```python
from build123d import *

# Parameters (mm, degrees)
SKETCH2_R           = 7.5
BOSS_EXTRUDE1_DEPTH = 15
SKETCH3_R           = 6.5
BOSS_EXTRUDE2_DEPTH = 7.5
SKETCH4_R           = 11
BOSS_EXTRUDE3_DEPTH = 15
SKETCH5_R           = 20
CUT_EXTRUDE1_DEPTH  = 235


with BuildPart() as part:
    # Sketch1 → Revolve1 (revolve)
    with BuildSketch(Plane.XY, mode=Mode.PRIVATE) as revolve1_sk:
        Polygon((0, 0), (35, 0), (35, 50), (30, 50), (30, 130), (35, 130), (35, 180), (22.65711135, 250), (30, 250), (30, 260), (0, 260), align=None)
    revolve(revolve1_sk.sketch.rotate(Axis((0, 0, 0), (0, 1, 0)), 90), axis=Axis((0, 0, 0), (0, 1, 0)))

    # Sketch2 → Boss-Extrude1 (add)
    with BuildSketch(Plane.XY.offset(35)):
        with BuildLine():
            Line((0, 0), (48, 0))
            Line((48, 0), (65, 0))
            ThreePointArc((65, 0), (79.305754261, 10.489413007), (73.603646545, 27.287280664))
            Line((73.603646545, 27.287280664), (41.166521698, 50))
            Line((41.166521698, 50), (0, 50))
            Line((0, 50), (0, 0))
        make_face()
        with Locations((48, 19)):
            Circle(SKETCH2_R, mode=Mode.SUBTRACT)
    boss_extrude1 = extrude(amount=-BOSS_EXTRUDE1_DEPTH)

    # Mirror1: Boss-Extrude1 across plane
    add(boss_extrude1.mirror(Plane.XY))

    # Sketch3 → Boss-Extrude2 (add, symmetric)
    with BuildSketch(Plane.XY):
        with BuildLine():
            Line((0, 180), (0, 140.71))
            Line((0, 140.71), (55, 140.71))
            Line((55, 140.71), (60, 140.71))
            ThreePointArc((60, 140.71), (71.563565439, 149.503139487), (66.180456899, 162.996007608))
            Line((66.180456899, 162.996007608), (37.881061244, 180))
            Line((37.881061244, 180), (0, 180))
        make_face()
        with Locations((55, 155)):
            Circle(SKETCH3_R, mode=Mode.SUBTRACT)
    boss_extrude2 = extrude(amount=BOSS_EXTRUDE2_DEPTH, both=True)

    # Mirror2: Boss-Extrude2 across plane
    add(boss_extrude2.mirror(Plane(origin=(0, 0, 0), x_dir=(0, 0, 1), z_dir=(1, 0, 0))))

    # Sketch4 → Boss-Extrude3 (add)
    with BuildSketch(Plane.XY.offset(5)):
        with BuildLine():
            Line((-20, 290), (-20, 258.467022151))
            Line((-20, 258.467022151), (20, 258.467022151))
            Line((20, 258.467022151), (20, 290))
            ThreePointArc((20, 290), (0, 310), (-20, 290))
        make_face()
        with Locations((0, 290)):
            Circle(SKETCH4_R, mode=Mode.SUBTRACT)
    extrude(amount=BOSS_EXTRUDE3_DEPTH)

    # Sketch5 → Cut-Extrude1 (cut)
    with BuildSketch(Plane.XZ):
        with Locations(Location((0, 0, 0), (0, 0, 270))):
            Circle(SKETCH5_R)
    extrude(amount=-CUT_EXTRUDE1_DEPTH, mode=Mode.SUBTRACT)


solid = part.part
```
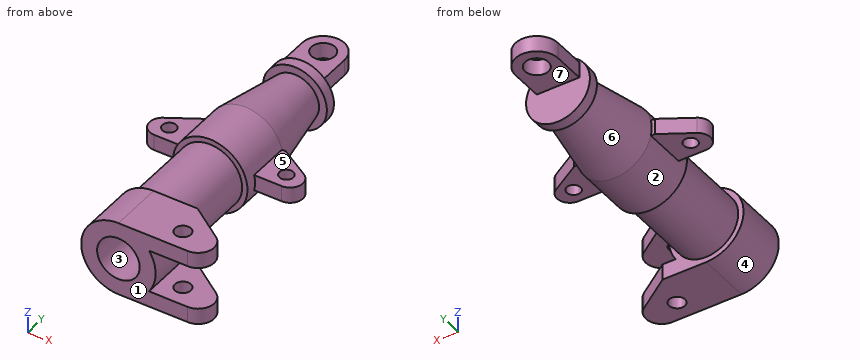
The listing builds one solid part. Answer for the finished solid, in the listing's coordinates (mm). Face numbers are marked on the shaded views. A direction names the side the tool comes from. Coordinates: 2 decimals unless noted, no trailing zeros. Loops run counter-clockwise (first coordinate to the right, second up) from the corner with the lowest first, then second, coordinate; pieces in that order, holes last. Notation, with made-up numbers: M -15,14 L 44,14 A28 cw 44,33 Z; hole C -25.75,71.5 d11. An arc over 180 degrees is marked long. Answer as a JSON object with one key per item and string values. Group by question number.
Item 1: Section C-C (y = 43) is taken. Write down the section's boundary in (x, z).
Item 2: Determine the mould class of the marked faces 1, 2, 3 and 4 for opening direction X: +X half, -X half, draft (parallel to the pull), parting line (faces both ways), or undercut.
Item 3: Which of the six approach directions +Z, -Z, +X, -X, +Y, -Y give full straight-line access (tool end or side, diameter ignored) to the marked faces 5, 6 and 7?
Item 4: Section D-D (z = -26.5) is taken. Give the number of separate pieces and of enclosed holes in the cut face, and give its area (3 significant figures).
Item 5: Each of these flat-tipped pins is pushed along its axis until it touches: P1, Ø1.1, axis at x = -35.5, z = 3.5, coming from the +Y side; P2, Ø5, axis at x = 38.5, y = 159.5, coming from the -Z side; P3, Ø10, axis at y = 209, z = 16, coming from the +X side. Where does it stop, or does it pass through?
Item 6: Section A-A (y = 155) is taken. Write down the section's boundary in (x, z).
Item 7: Section B-B (x = -55) is taken. Write down the section's boundary in (y, z).
Item 8: Consider L1, parallel to X at y = 93, z = 0; L2, parallel to Z at x = 11, y = 294.5; L3, parallel to X at y = 15, z = -23.5. Determine where each line is inside the solid, lowest interval first.
Solved:
{
 "1": {"outline": "M 0,-35 L 51.16,-35 L 51.16,-20 L 28.72,-20 A35 ccw 28.72,20 L 51.16,20 L 51.16,35 L 0,35 A35 ccw Z; hole C 0,0 d40"},
 "2": {"face 1": "draft", "face 2": "parting line", "face 3": "undercut", "face 4": "-X half"},
 "3": {"face 5": "+Z, +X, +Y, -Y", "face 6": "none", "face 7": "-Z, +X, -X, +Y"},
 "4": {"separate pieces": "2", "enclosed holes": "1", "area": "10,600 mm2"},
 "5": {"P1": "stops at y = 180", "P2": "stops at z = -7.5", "P3": "stops at x = 28"},
 "6": {"outline": "M -71.78,-7.5 L -61.5,-7.5 L -61.5,7.5 L -71.78,7.5 Z; M -48.5,-7.5 L -34.19,-7.5 A35 ccw 34.19,-7.5 L 48.5,-7.5 L 48.5,7.5 L 34.19,7.5 A35 ccw -34.19,7.5 L -48.5,7.5 Z; M 61.5,-7.5 L 71.78,-7.5 L 71.78,7.5 L 61.5,7.5 Z; hole C 0,0 d40"},
 "7": {"outline": "M 140.71,-7.5 L 148.5,-7.5 L 148.5,7.5 L 140.71,7.5 Z; M 161.5,-7.5 L 169.71,-7.5 L 169.71,7.5 L 161.5,7.5 Z"},
 "8": {"L1": "x = -30 to -20, 20 to 30", "L2": "z = 5 to 20", "L3": "x = -25.94 to 41.66, 54.34 to 80"}
}
